from build123d import *

# Parameters (mm, degrees)
CUBE003_W                     = 500
CUBE003_H                     = 500
CUBE003_DEPTH                 = 500
CYLINDER006_R                 = 2.25
CYLINDER006_DEPTH             = 1000
CYLINDER005_R                 = 2.25
CYLINDER005_DEPTH             = 1000
CYLINDER004_R                 = 7.25
CYLINDER004_DEPTH             = 6.5
CYLINDER003_R                 = 7.25
CYLINDER003_DEPTH             = 6.5
GROUP003_PLACEMENT_ANGLE      = 180
CYLINDER002_R                 = 7.25
CYLINDER002_DEPTH             = 6.5
CYLINDER001_R                 = 7.25
CYLINDER001_DEPTH             = 6.5
CYLINDER_R                    = 4
CYLINDER_DEPTH                = 200
CUBE002_W                     = 60
CUBE002_H                     = 21
CUBE002_DEPTH                 = 21
CUBE001_W                     = 30
CUBE001_H                     = 31
CUBE001_DEPTH                 = 26
DIFFERENCE002_PITCH_ANGLE     = 90
DIFFERENCE002_PLACEMENT_ANGLE = 90
REFINELINEAREXTRUDE_R         = 12
REFINELINEAREXTRUDE_R_2       = 1.675
LINEAREXTRUDE_DEPTH           = 20
CUBE_W                        = 42.3
CUBE_H                        = 42.3
CUBE_DEPTH                    = 5


with BuildPart() as cube003:
    # cube003 → cube003 (new body)
    with BuildSketch(Plane(origin=(-250, -510, -250), x_dir=(1, 0, 0), z_dir=(0, 0, 1))):
        with Locations((250, 250)):
            Rectangle(CUBE003_W, CUBE003_H)
    extrude(amount=CUBE003_DEPTH)


with BuildPart() as cylinder006:
    # cylinder006 → cylinder006 (new body)
    with BuildSketch(Plane(origin=(15.5, 500, 0), x_dir=(1, 0, 0), z_dir=(0, -1, 0))):
        Circle(CYLINDER006_R)
    extrude(amount=CYLINDER006_DEPTH)


with BuildPart() as union002:
    # cylinder005 → cylinder005 (new body)
    with BuildSketch(Plane.XZ.offset(-500)):
        Circle(CYLINDER005_R)
    extrude(amount=CYLINDER005_DEPTH)

    # Group005: union cylinder006
    add(cylinder006.part)


with BuildPart() as union002_1:
    # Group005 placement: moved
    add(union002.part.moved(Location((2.25, 0, -15.5))))

    # union002: union cube003
    add(cube003.part)


with BuildPart() as cylinder004:
    # cylinder004 → cylinder004 (new body)
    with BuildSketch(Plane(origin=(15.5, 0, 0), x_dir=(1, 0, 0), z_dir=(0, -1, 0))):
        Circle(CYLINDER004_R)
    extrude(amount=CYLINDER004_DEPTH)


with BuildPart() as group003:
    # cylinder003 → cylinder003 (new body)
    with BuildSketch(Plane.XZ):
        Circle(CYLINDER003_R)
    extrude(amount=CYLINDER003_DEPTH)

    # Group003: union cylinder004
    add(cylinder004.part)


with BuildPart() as group003_1:
    # Group003 placement: moved
    add(group003.part.moved(Location((2.25, 10.5, -15.5))).rotate(Axis((2.25, 10.5, -15.5), (1, 0, 0)), GROUP003_PLACEMENT_ANGLE))


with BuildPart() as cylinder002:
    # cylinder002 → cylinder002 (new body)
    with BuildSketch(Plane(origin=(15.5, 0, 0), x_dir=(1, 0, 0), z_dir=(0, -1, 0))):
        Circle(CYLINDER002_R)
    extrude(amount=CYLINDER002_DEPTH)


with BuildPart() as group004:
    # cylinder001 → cylinder001 (new body)
    with BuildSketch(Plane.XZ):
        Circle(CYLINDER001_R)
    extrude(amount=CYLINDER001_DEPTH)

    # Group002: union cylinder002
    add(cylinder002.part)


with BuildPart() as group004_1:
    # Group002 placement: moved
    add(group004.part.moved(Location((2.25, -10.5, -15.5))))

    # Group004: union Group003
    add(group003_1.part)


with BuildPart() as cylinder:
    # cylinder → cylinder (new body)
    with BuildSketch(Plane(origin=(-100, 15, 13), x_dir=(0, 1, 0), z_dir=(1, 0, 0))):
        Circle(CYLINDER_R)
    extrude(amount=CYLINDER_DEPTH)


with BuildPart() as union:
    # cube002 → cube002 (new body)
    with BuildSketch(Plane(origin=(-30, -10.5, -13), x_dir=(1, 0, 0), z_dir=(0, 0, 1))):
        with Locations((30, 10.5)):
            Rectangle(CUBE002_W, CUBE002_H)
    extrude(amount=CUBE002_DEPTH)

    # union: union cylinder
    add(cylinder.part)


with BuildPart() as difference002:
    # cube001 → cube001 (new body)
    with BuildSketch(Plane(origin=(-15, -15.5, -13), x_dir=(1, 0, 0), z_dir=(0, 0, 1))):
        with Locations((15, 15.5)):
            Rectangle(CUBE001_W, CUBE001_H)
    extrude(amount=CUBE001_DEPTH)

    # difference001: cut union
    add(union.part, mode=Mode.SUBTRACT)


with BuildPart() as difference002_1:
    # difference001 placement: moved
    add(difference002.part.moved(Location((10, 0, -13))))

    # union001: union Group004
    add(group004_1.part)

    # difference002: cut union002
    add(union002_1.part, mode=Mode.SUBTRACT)


with BuildPart() as difference002_2:
    # difference002 pitch: moved
    add(difference002_1.part.rotate(Axis((0, 0, 0), (0, 1, 0)), DIFFERENCE002_PITCH_ANGLE))


with BuildPart() as difference002_3:
    # difference002 placement: moved
    add(difference002_2.part.moved(Location((21.15, 5, 25))).rotate(Axis((21.15, 5, 25), (0, 0, 1)), DIFFERENCE002_PLACEMENT_ANGLE))


with BuildPart() as linearextrude:
    # RefineLinearExtrude → LinearExtrude (new body)
    with BuildSketch(Plane(origin=(0, 0, 0), x_dir=(0, 1, 0), z_dir=(0, 0, 1))):
        Circle(REFINELINEAREXTRUDE_R)
        with Locations((15.5, -15.5)):
            Circle(REFINELINEAREXTRUDE_R_2)
        with Locations((15.5, 15.5)):
            Circle(REFINELINEAREXTRUDE_R_2)
        with Locations((-15.5, 15.5)):
            Circle(REFINELINEAREXTRUDE_R_2)
        with Locations((-15.5, -15.5)):
            Circle(REFINELINEAREXTRUDE_R_2)
    extrude(amount=LINEAREXTRUDE_DEPTH)


with BuildPart() as linearextrude_1:
    # LinearExtrude placement: moved
    add(linearextrude.part.moved(Location((21.15, 21.15, -10))))


with BuildPart() as group006:
    # cube → cube (new body)
    with BuildSketch(Plane.XY):
        with Locations((21.15, 21.15)):
            Rectangle(CUBE_W, CUBE_H)
    extrude(amount=CUBE_DEPTH)

    # difference: cut LinearExtrude
    add(linearextrude_1.part, mode=Mode.SUBTRACT)

    # Group006: union difference002
    add(difference002_3.part)


solid = group006.part
Check sheet for the modelled part. Datum: model origin and axes. Units: mm. A direction names the side the tool comes from. Round coordinates to 2 decimals unless told otherwise and drop trailing zeros. Loops run counter-clockwise (first coordinate to the right, second up) from the corner with the lowest first, then second, coordinate; pieces in that order, holes last. Notation, with made-up numbers: (47, 63.5) - (102, 63.5) arc R13 cw to (102, 75.5) - close; hole circle Ø6 at (45, 36.25). An arc over 180 degrees is marked (long way). Answer as CSV lines item,"result". Start each with the question number.
Item 1: Depth check by flat-ended pin: P1, Ø1.5, axis at y = 2, z = 23, coming from the +X side; P2, Ø15, axis at x = 32.5, z = 9, coming from the -Y side; P3, Ø5.5, axis at x = 5.65, y = 5.65, coming from the +Z side. Enter the tip coordinate at first touch or a pass-through.
Item 2: Section check A-A (y = 21.15). Record the boundary of the cut face in (x, z).
Item 3: Set-up check for faces 4 (the cylindrical face through (4.91, -17.69, 8.19)), 5 (the flat face through (31.15, 2, 18)), 6 (the flat face through (21, 5, 18)), 7 (the flat face through (3, 0, 2)), 8 (the flat face through (23, 0, 15)): record each of +Z, -Z, +X, -X, +Y, -Y from which the full face is reachable in a straight line by a thin tool's end or side.
Item 4: Release check for a two-part mould opening along X. For faces 1 (the flat face through (4.15, -12.2, 9)), 2 (the cylindrical face through (6.29, 38.2, 2.46)), 3 (the flat face through (10.65, -11, 15)) record: +X half, -X half, draft (parallel to the pull), parting line (faces both ways), or undercut.
Item 5: Section check B-B (x = 36.65). Record the boundary of the cut face in (y, z) (3 decimals), and give its area (3 significant figures).
Item 6: Scan lines: line 1 (Z direction, x = 9, y = -10); line 2 (Y direction, x = 6.25, z = 7.25); line 3 (X direction, y = -5, z = 23.5). Record each from-to range of solid material in increasing order. Write a range as [from, to].
Item 7: Section check C-C (z = 22.75). Record the boundary of the cut face in (x, y), and give its area (3 significant figures).
Item 8: Section check D-D (x = 21.15). Record the boundary of the cut face in (y, z).
Report:
1,P1,"stops at x = 31.15"
1,P2,"stops at y = 0"
1,P3,"stops at z = 5"
2,outline,"(0, 0) - (9.15, 0) - (9.15, 5) - (0, 5) - close; (33.15, 0) - (42.3, 0) - (42.3, 5) - (33.15, 5) - close"
3,face 4,"-X"
3,face 5,"+Z, +X, +Y, -Y"
3,face 6,"+Z, +X, -X, +Y"
3,face 7,"+Z, -Z, -X"
3,face 8,"+Z, -Z, +X, -Y"
4,face 1,"-X half"
4,face 2,"undercut"
4,face 3,"+X half"
5,outline,"(0, 0) - (3.975, 0) - (3.975, 5) - (0, 5) - close; (7.325, 0) - (34.975, 0) - (34.975, 5) - (7.325, 5) - close; (38.325, 0) - (42.3, 0) - (42.3, 5) - (38.325, 5) - close"
5,area,"178 mm2"
6,line 1,"z = [0, 5.06], [9.44, 20.56], [24.94, 30]"
6,line 2,"y = [-21, -12.75], [-8.25, 1]"
6,line 3,"x = [4.15, 10.65]"
7,outline,"(4.15, -17.75) - (5.65, -17.75) - (5.65, -21) - (10.65, -21) - (10.65, -12.75) - (4.15, -12.75) - close; (4.15, -8.25) - (10.65, -8.25) - (10.65, 0) - (31.15, 0) - (31.15, 5) - (10.15, 5) arc R4 cw to (5.65, 1.03) - (5.65, -3.25) - (4.15, -3.25) - close"
7,area,"210 mm2"
8,outline,"(0, 0) - (9.15, 0) - (9.15, 5) - (5, 5) - (5, 30) - (0, 30) - close; (33.15, 0) - (42.3, 0) - (42.3, 5) - (33.15, 5) - close"
